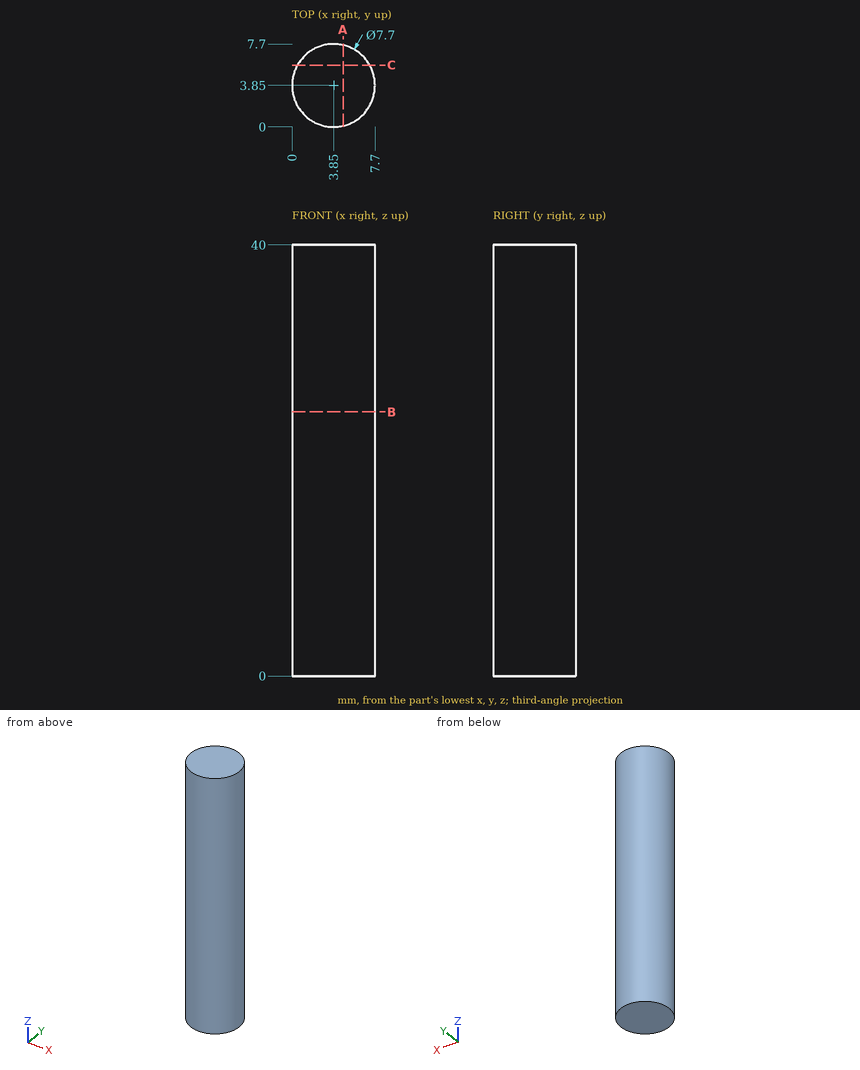
Verification items for this drawing (mm, ordinates from the low corner). Coordinates: 2 decimals unless noted, no trailing zeros. Write each loop counter-clockwise with the first axis right and the second up, starting at its lowest first coordinate (ties: lowest second). Pieces come first, ordered by that corner, then holes. Notation, with made-up numbers: M -40,34 L -31,34 A7 ccw -31,46 Z; hole C 17,-21.5 d7. An arc over 180 degrees is marked long. Use one line per item in the form item = value. Start each with the question number.
1) Section check B-B on z = 24.5. Enter the section's corners in (x, y).
2) Section check A-A on x = 4.75. Enter the section's corners in (y, z).
3) Go/stop test with flat-tipped pins: pin 1 Ø1 at (y, z) = (1.5, 30.5) entering from +X; pin 2 Ø3 at (x, z) = (6.5, 16.5) entering from +Y; pin 3 Ø1.5 at (x, z) = (1, 20.5) entering from -Y. Record where each tip stops, or that it passes through.
4) Thickness scan on probe 1 along Y at (x, z) = (4, 21); probe 2 along X at (y, z) = (5, 26.5). Record the ranges inside material, lowest first. Write a range as from..to.
5) Section check C-C on y = 5.75. Enter the section's corners in (x, z), and give its area (3 significant figures).
Responses:
q1.outline = C 3.85,3.85 d7.7
q2.outline = M 0.11,0 L 7.59,0 L 7.59,40 L 0.11,40 Z
q3.pin_1 = 7.23
q3.pin_2 = 7.52
q3.pin_3 = 0.62
q4.probe_1 = 0..7.7
q4.probe_2 = 0.18..7.52
q5.outline = M 0.5,0 L 7.2,0 L 7.2,40 L 0.5,40 Z
q5.area = 268 mm2
